```python
from build123d import *

# Parameters (mm, degrees)
SKETCH_1_R           = 90
EXTRUDE_1_DEPTH      = 10
SKETCH_2_R           = 70
EXTRUDE_2_DEPTH      = 10
SKETCH_4_R           = 80
SKETCH_4_R_2         = 46.5
EXTRUDE_3_DEPTH      = 21.15
EXTRUDE_4_REACH      = 226.555
EXTRUDE_4_END_RADIUS = 80
SKETCH_5_W           = 100
SKETCH_5_H           = 42.3
FILLET_1_R           = 10
SKETCH_6_R           = 46.5
CUT_EXTRUDE_1_DEPTH  = 1


with BuildPart() as part:
    # Sketch 1 → Extrude 1 (new body)
    with BuildSketch(Plane(origin=(0, 0, 0), x_dir=(1, 0, 0), z_dir=(0, 1, 0))):
        with Locations(Location((0, 0, 0), (0, 0, 270))):
            Circle(SKETCH_1_R)
    extrude(amount=EXTRUDE_1_DEPTH)

    # Sketch 2 → Extrude 2 (add)
    with BuildSketch(Plane(origin=(0, 10, 0), x_dir=(1, 0, 0), z_dir=(0, 1, 0))):
        with Locations(Location((0, 0, 0), (0, 0, 270))):
            Circle(SKETCH_2_R)
    extrude(amount=EXTRUDE_2_DEPTH)



with BuildPart() as body_2:
    # Sketch 4 → Extrude 3 (new, symmetric)
    with BuildSketch(Plane.XY):
        with Locations((0, 125)):
            Circle(SKETCH_4_R)
        with Locations((0, 125)):
            Circle(SKETCH_4_R_2, mode=Mode.SUBTRACT)
    extrude(amount=EXTRUDE_3_DEPTH, both=True)


with BuildPart() as part_1:
    add(part.part)

    add(body_2.part)  # Extrude 4 merges body 2
    # Extrude 4: up to this cylinder (the profile starts outside it)
    extrude_4_end = Plane(origin=(0, 125, 0), z_dir=(0, 0, -1)) * Cylinder(EXTRUDE_4_END_RADIUS, 614.11, mode=Mode.PRIVATE)
    # Sketch 5 → Extrude 4 (add, up to the surface)
    with BuildSketch(Plane(origin=(0, 20, 0), x_dir=(1, 0, 0), z_dir=(0, 1, 0)), mode=Mode.PRIVATE) as extrude_4_sk1:
        Rectangle(SKETCH_5_W, SKETCH_5_H)
    extrude_4_tool1 = extrude(extrude_4_sk1.sketch, amount=EXTRUDE_4_REACH, mode=Mode.PRIVATE) - extrude_4_end
    add(extrude_4_tool1.solids().sort_by_distance((0, 20, 0))[0])

    # Fillet 1
    fillet_1_edges = [part_1.edges().sort_by_distance(p)[0] for p in [
        (50, 41.275010008, -21.15),
        (50, 41.275010008, 21.15),
        (-50, 41.275010008, -21.15),
        (-50, 41.275010008, 21.15),
    ]]
    fillet(fillet_1_edges, radius=FILLET_1_R)

    # Sketch 6 → Cut-Extrude 1 (cut)
    with BuildSketch(Plane.XZ):
        with Locations(Location((0, 0, 0), (0, 0, 270))):
            Circle(SKETCH_6_R)
    extrude(amount=-CUT_EXTRUDE_1_DEPTH, mode=Mode.SUBTRACT)


solid = part_1.part
```
The model under review builds one solid part; all positions refer to its coordinate system, in mm. A direction names the side the tool comes from. Round coordinates to 2 decimals unless told otherwise and drop trailing zeros. Loops run counter-clockwise (first coordinate to the right, second up) from the corner with the lowest first, then second, coordinate; pieces in that order, holes last.
Item 1: Take a section at A-A (z = 0). Write out the cut boundary in (x, y), then the cut area to 3 significant figures.
Determined:
outline: (-90, 0) - (-46.5, 0) - (-46.5, 1) - (46.5, 1) - (46.5, 0) - (90, 0) - (90, 10) - (70, 10) - (70, 20) - (50, 20) - (50, 62.55) arc R80 ccw (long way) to (-50, 62.55) - (-50, 20) - (-70, 20) - (-70, 10) - (-90, 10) - close; hole circle Ø93 at (0, 125)
area: 19,500 mm2
Item 2: For faces 1 (the face through (50, 41, 0)), 2 (the face through (46.1, 0.5, 6.1)), 3 (the face through (-47.15, 41.57, 18.14)), list the 3-axis set-ups (+Z, -Z, +X, -X, +Y, -Y) from which the entire face can be reached by the end or side of a thin tool; tool diameter is ignored.
Determined:
face 1: +Z, -Z, +X
face 2: -Y
face 3: +Z, -X
Item 3: Take a section at C-C (x = 0). Write out the cut boundary in (y, z).
Determined:
outline: (0, -90) - (10, -90) - (10, -70) - (20, -70) - (20, -21.15) - (78.5, -21.15) - (78.5, 21.15) - (20, 21.15) - (20, 70) - (10, 70) - (10, 90) - (0, 90) - (0, 46.5) - (1, 46.5) - (1, -46.5) - (0, -46.5) - close; (171.5, -21.15) - (205, -21.15) - (205, 21.15) - (171.5, 21.15) - close
Item 4: Mouldability with a two-part tool opening along Y and no side actions: class faces 4 (the face through (1, 1, 1)), 5 (the face through (-34.471, 4.93, 83.137)), 6 (the face through (-50, 41, 0)) as released by +Y, released by -Y, zero draft, split by the parting line, or undercut.
Determined:
face 4: released by -Y
face 5: zero draft
face 6: undercut
Item 5: Take a section at B-B (y = 125). Write out the cut boundary in (x, z).
Determined:
outline: (-80, -21.15) - (-46.5, -21.15) - (-46.5, 21.15) - (-80, 21.15) - close; (46.5, -21.15) - (80, -21.15) - (80, 21.15) - (46.5, 21.15) - close
Item 6: Take a section at D-D (y = 40.5). Write out the cut boundary in (x, z).
Determined:
outline: (-50, -11.15) arc R10 ccw to (-40, -21.15) - (40, -21.15) arc R10 ccw to (50, -11.15) - (50, 11.15) arc R10 ccw to (40, 21.15) - (-40, 21.15) arc R10 ccw to (-50, 11.15) - close
Item 7: Clearance check with flat-ended pins moving along their axes: pin 1 Ø3 at (x, z) = (55, 33.5) entering from +Y; pin 2 Ø11 at (y, z) = (41, -0.5) entering from -X; pin 3 Ø6 at (y, z) = (74, 17) entering from -X. State where each tip first meets the part, or that it passes through.
Determined:
pin 1: stops at y = 20
pin 2: stops at x = -50
pin 3: stops at x = -64
Item 8: For line 1 (Y direction, x = 0, z = 10.5); line 2 (X direction, y = 41, z = 1); line 3 (Z direction, x = -30, y = 52.5), list the stretches that pass through material, from the lowest coordinate up.
Determined:
line 1: y = 1 to 78.5, 171.5 to 205
line 2: x = -50 to 50
line 3: z = -21.15 to 21.15
